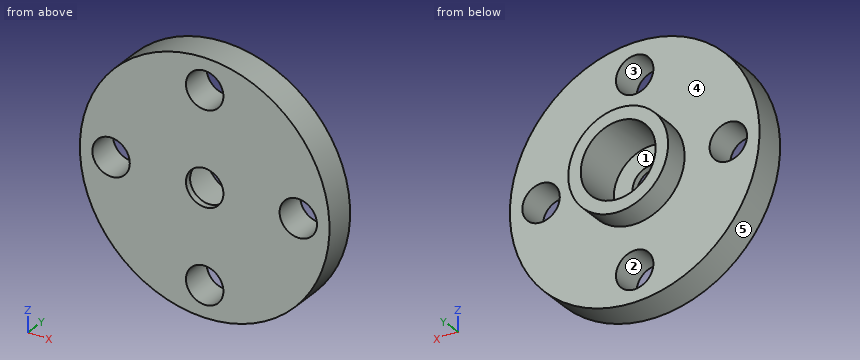
```python
from build123d import *

# Parameters (mm, degrees)
SKETCH2_R          = 1.5
CUT_EXTRUDE1_DEPTH = 10


with BuildPart() as part:
    # Sketch1 → Revolve1 (revolve)
    with BuildSketch(Plane.XY, mode=Mode.PRIVATE) as revolve1_sk:
        Polygon((3, 0), (4, 0), (4, -2), (10, -2), (10, -4.5), (1.5, -4.5), (1.5, -4), (3, -4), align=None)
    revolve(revolve1_sk.sketch.rotate(Axis((0, 3.424478083, 0), (0, -1, 0)), 90), axis=Axis((0, 3.424478083, 0), (0, -1, 0)))

    # Sketch2 → Cut-Extrude1 (cut)
    with BuildSketch(Plane.XZ.offset(4.5)):
        with Locations(Location((0, -7.5, 0), (0, 0, 270))):
            Circle(SKETCH2_R)
        with Locations(Location((-7.5, 0, 0), (0, 0, 270))):
            Circle(SKETCH2_R)
        with Locations(Location((0, 7.5, 0), (0, 0, 270))):
            Circle(SKETCH2_R)
        with Locations(Location((7.5, 0, 0), (0, 0, 270))):
            Circle(SKETCH2_R)
    extrude(amount=-CUT_EXTRUDE1_DEPTH, mode=Mode.SUBTRACT)


solid = part.part
```
The listing builds one solid part. Answer for the finished solid, in the listing's coordinates (mm). Face numbers are marked on the shaded views. A direction names the side the tool comes from. Coordinates: 2 decimals unless noted, no trailing zeros. Order: outer loops, then holes, each group sorted by start corner. A loop starts at its lowest first (then second) coordinate and runs counter-clockwise, first axis right, second up. Notation, with made-up numbers: M -24,86 L 6,86 A26 ccw 6,102 Z; hole C 87,8 d7. An arc over 180 degrees is marked long. Answer as a JSON object with one key per item and string values. Group by question number.
1. Flat-ended cylindrical pins translate along their axes: P1, Ø2.5, axis at x = 0, z = 0, coming from the +Y side; P2, Ø2, axis at x = -5.5, z = -1, coming from the +Y side; P3, Ø1.8, axis at x = 1, z = -1, coming from the +Y side; P4, Ø2, axis at y = -2, z = 2.5, coming from the +X side. Find the tip coordinate at first contact, or state that the pin passes through.
2. Section A-A on x = 0 is taken. Write down the section's boundary in (y, z).
3. Section D-D on z = -7.5 is taken. Write down the section's boundary in (x, y).
4. Straight lines are drawn through the part: line 1 (X direction, y = -4.4, z = 0); line 2 (X direction, y = -1.35, z = 0); line 3 (Z direction, x = -7.75, y = -2.75). For each, find the intervals that lie inside material, in ascending order.
5. Section C-C on y = -2.55 is taken. Write down the section's boundary in (x, z), then the cut area to 3 significant figures.
6. Section B-B on z = 0 is taken. Write down the section's boundary in (x, y), then the cut area to 3 significant figures.
7. Determine the mould class of the marked faces 3, 4 and 5 for opening direction X: released by +X, released by -X, zero draft, split by the parting line, or undercut.
8. A tool of negligible diameter and unlimited length cuts with its end or side. For the marked faces 1 and 2, from which of +Z, -Z, +X, -X, +Y, -Y can it reach the whole face along a straight path? Write none if from no direction.
Values follow:
{
 "1": {"P1": "through", "P2": "y = -2", "P3": "y = -4", "P4": "x = 9.89"},
 "2": {"outline": "M -4.5,-10 L -2,-10 L -2,-9 L -4.5,-9 Z; M -4.5,-6 L -2,-6 L -2,-4 L 0,-4 L 0,-3 L -4,-3 L -4,-1.5 L -4.5,-1.5 Z; M -4.5,1.5 L -4,1.5 L -4,3 L 0,3 L 0,4 L -2,4 L -2,6 L -4.5,6 Z; M -4.5,9 L -2,9 L -2,10 L -4.5,10 Z"},
 "3": {"outline": "M -6.61,-4.5 L -1.5,-4.5 L -1.5,-2 L -6.61,-2 Z; M 1.5,-4.5 L 6.61,-4.5 L 6.61,-2 L 1.5,-2 Z"},
 "4": {"line 1": "-10 to -9, -6 to -1.5, 1.5 to 6, 9 to 10", "line 2": "-4 to -3, 3 to 4", "line 3": "-6.32 to -1.48, 1.48 to 6.32"},
 "5": {"outline": "C 0,0 d20; hole C -7.5,0 d3; hole C 0,0 d6; hole C 0,-7.5 d3; hole C 0,7.5 d3; hole C 7.5,0 d3", "area": "258 mm2"},
 "6": {"outline": "M -10,-4.5 L -9,-4.5 L -9,-2 L -10,-2 Z; M -6,-4.5 L -1.5,-4.5 L -1.5,-4 L -3,-4 L -3,0 L -4,0 L -4,-2 L -6,-2 Z; M 1.5,-4.5 L 6,-4.5 L 6,-2 L 4,-2 L 4,0 L 3,0 L 3,-4 L 1.5,-4 Z; M 9,-4.5 L 10,-4.5 L 10,-2 L 9,-2 Z", "area": "25.5 mm2"},
 "7": {"face 3": "undercut", "face 4": "zero draft", "face 5": "split by the parting line"},
 "8": {"face 1": "+Y", "face 2": "+Y, -Y"}
}
